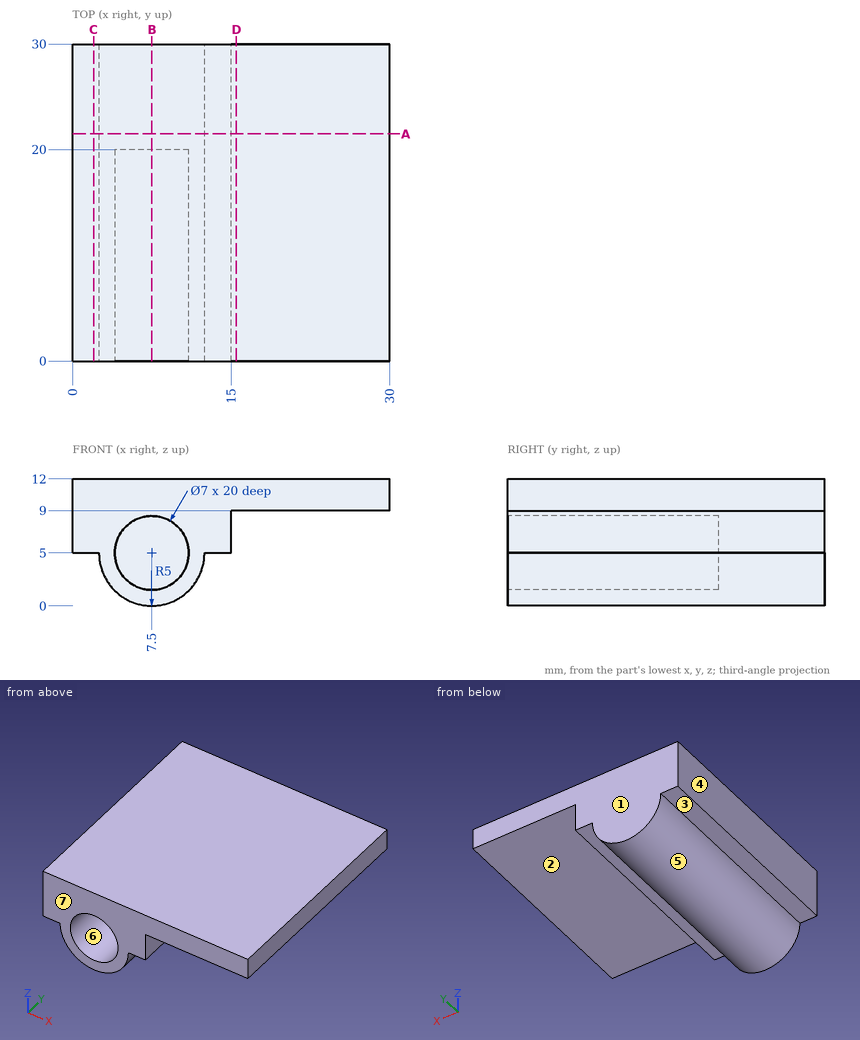
Source: three-view drawing plus pictorial views. Frame: mm from the lowest corner of the part. A direction names the side the tool comes from. Give positions to 0.01 mm unless a question says otherwise; leave off trailing zeros. Loops run counter-clockwise (first coordinate to the right, second up) from the corner with the lowest first, then second, coordinate; pieces in that order, holes last. Notation, with made-up numbers: (0, -32.75) -> (32, -32.75) arc R21 ccw to (32, -11.75) -> close; hole circle Ø5 at (9.5, -25.5). An arc over 180 degrees is marked (long way). Use a Markdown table: item, result. Add a question column.
(1) Access query for the marked faces 1, 2 and 3. Directions: +Z, -Z, +X, -X, +Y, -Y. A direction counts if a zero-diameter tool reaches every point of the face in a straight line with its end or side. Return the directions, or none.
(2) Section query B-B (x = 7.5). Output: boundary loops of the cut face in (y, z), then the cut area to 3 significant figures.
(3) First-contact query: pin 1 Ø3 at (x, y) = (13.5, 7.5) entering from -Z; pin 2 Ø3 at (y, z) = (9.5, 2.5) entering from -X; pin 3 Ø4.5 at (x, y) = (22, 12) entering from -Z. Flat tips, straight axial feed; report the tip coordinate or a pass-through.
(4) Section query A-A (y = 21.5). Output: boundary loops of the cut face in (x, z), then the cut area to 3 significant figures.
(5) Section query D-D (x = 15.5). Output: boundary loops of the cut face in (y, z).
(6) Pull-direction query (X, two-part tool) for the marked faces 4, 5, 6 and 7; classes: +X half, -X half, draft (parallel to the pull), parting line (faces both ways), or undercut.
(7) Ray query, line 1 (Z direction, x = 7.5, y = 15.5); line 2 (Z direction, x = 18.25, y = 29.25); line 3 (Y direction, x = 10.25, z = 6.5). Return the intervals inside material, ascending.
(8) Section query C-C (x = 2). Output: boundary loops of the cut face in (y, z).
Checked values:
| question | item | result |
|---|---|---|
| 1 | face 1 | +Z, -Z, +X, -X, +Y |
| 1 | face 2 | -Z, +X, +Y, -Y |
| 1 | face 3 | -Z, -X, +Y, -Y |
| 2 | outline | (0, 0) -> (30, 0) -> (30, 12) -> (0, 12) -> (0, 8.5) -> (20, 8.5) -> (20, 1.5) -> (0, 1.5) -> close |
| 2 | area | 220 mm^2 |
| 3 | pin 1 | z = 2.82 |
| 3 | pin 2 | x = 2.6 |
| 3 | pin 3 | z = 9 |
| 4 | outline | (0, 5) -> (2.5, 5) arc R5 ccw to (12.5, 5) -> (15, 5) -> (15, 9) -> (30, 9) -> (30, 12) -> (0, 12) -> close |
| 4 | area | 189 mm^2 |
| 5 | outline | (0, 9) -> (30, 9) -> (30, 12) -> (0, 12) -> close |
| 6 | face 4 | -X half |
| 6 | face 5 | parting line |
| 6 | face 6 | undercut |
| 6 | face 7 | draft |
| 7 | line 1 | 0 to 1.5, 8.5 to 12 |
| 7 | line 2 | 9 to 12 |
| 7 | line 3 | 20 to 30 |
| 8 | outline | (0, 5) -> (30, 5) -> (30, 12) -> (0, 12) -> close |
